Check sheet for the modelled part. Datum: model origin and axes. Units: mm. Face numbers are marked on the shaded views. Coordinates: 2 decimals unless noted, no trailing zeros. Loops run counter-clockwise (first coordinate to the right, second up) from the corner with the lowest first, then second, coordinate; pieces in that order, holes last. Notation, with made-up numbers: M 76,85.25 L 82,85.25 A8 ccw 82,95.25 Z; hole C 25.5,14.25 d6. An arc over 180 degrees is marked long. Answer in a Markdown table with one row per item. Add a question column.
```python
from build123d import *

# Parameters (mm, degrees)
SKETCH_1_R                = 60
EXTRUDE_1_DEPTH           = 10
SKETCH_4_R                = 30
CUT_EXTRUDE_1_DEPTH       = 86.440037453
HOLE_WIZARD_1_D           = 4.5
HOLE_WIZARD_1_CBORE_D     = 8
HOLE_WIZARD_1_CBORE_DEPTH = 4.6
PATTERN_CIRCULAR_1_COUNT  = 16
HOLE_WIZARD_2_D           = 5.5
HOLE_WIZARD_2_CBORE_D     = 10
HOLE_WIZARD_2_CBORE_DEPTH = 5.7
PATTERN_CIRCULAR_2_COUNT  = 10


with BuildPart() as part:
    # 草图1 → 凸台-拉伸1 (new body)
    with BuildSketch(Plane.XY):
        Circle(SKETCH_1_R)
    extrude(amount=EXTRUDE_1_DEPTH)

    # 草图4 → 切除-拉伸1 (cut, through all)
    with BuildSketch(Plane.XY.offset(10)):
        Circle(SKETCH_4_R)
    extrude(amount=-CUT_EXTRUDE_1_DEPTH, mode=Mode.SUBTRACT)

    # 打孔尺寸(%根据)内六角圆柱头螺钉的类型1 (through all)
    with Locations(Plane.XY.offset(10)):
        with Locations((0, 38.5)):
            hole_wizard_1 = CounterBoreHole(HOLE_WIZARD_1_D / 2, HOLE_WIZARD_1_CBORE_D / 2, HOLE_WIZARD_1_CBORE_DEPTH)

    # 阵列(圆周)1: 打孔尺寸(%根据)内六角圆柱头螺钉的类型1 ×16 about axis
    pattern_circular_1_axis = Axis((0, 0, 0), (0, 0, 1))
    for i in range(1, PATTERN_CIRCULAR_1_COUNT):
        add(hole_wizard_1.rotate(pattern_circular_1_axis, i * 360 / PATTERN_CIRCULAR_1_COUNT), mode=Mode.SUBTRACT)

    # 打孔尺寸(%根据)内六角圆柱头螺钉的类型2 (through all)
    with Locations(Plane(origin=(0, 0, 0), x_dir=(-1, 0, 0), z_dir=(0, 0, -1))):
        with Locations((0, 52.5)):
            hole_wizard_2 = CounterBoreHole(HOLE_WIZARD_2_D / 2, HOLE_WIZARD_2_CBORE_D / 2, HOLE_WIZARD_2_CBORE_DEPTH)

    # 阵列(圆周)2: 打孔尺寸(%根据)内六角圆柱头螺钉的类型2 ×10 about axis
    pattern_circular_2_axis = Axis((0, 0, 0), (0, 0, 1))
    for i in range(1, PATTERN_CIRCULAR_2_COUNT):
        add(hole_wizard_2.rotate(pattern_circular_2_axis, i * 360 / PATTERN_CIRCULAR_2_COUNT), mode=Mode.SUBTRACT)


solid = part.part
```
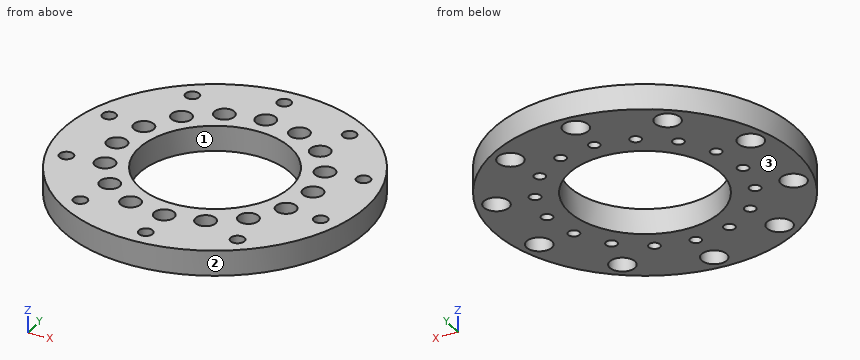
Q1. Mould release check, pull along Y, two halves, no side actions. Record for the marked faces 1, 2 and 3: released by +Y, released by -Y, zero draft, split by the parting line, or undercut.
Q2. Cross-section at C-C (y = -52.5). Record the cut outline in (x, z), plus the area to 3 significant figures.
Q3. Thickness scan on L1, parallel to Y at x = 0, z = 8.9; L2, parallel to Y at x = 0, z = 1.65; L3, parallel to Y at x = 51.5, z = 2.25. Record the ranges inside material, lowest first.
Q4. Go/stop test with flat-tipped pins: pin 1 (6 mm diameter, centred on y = -0.5, z = 9, fed in from +X); pin 2 (3 mm diameter, centred on x = 25.5, z = 4.5, fed in from -Y); pin 3 (1 mm diameter, centred on x = -42, z = 3.5, fed in from +Y); pin 4 (3.5 mm diameter, centred on x = 27.22, y = 27.22, fed in from +Z). Record where each tip stops, or that it passes through.
Q5. Cross-section at B-B (x = 0). Count the separate pieces of the cut face and the enclosed holes in it, plus the area to 4 significant figures.
Q6. Cross-section at A-A (y = 0). Record the cut outline in (x, z), plus the area to 3 significant figures.
Answer key:
| question | item | result |
|---|---|---|
| 1 | face 1 | undercut |
| 1 | face 2 | split by the parting line |
| 1 | face 3 | zero draft |
| 2 | outline | M -29.05,0 L -5,0 L -5,5.7 L -2.75,5.7 L -2.75,10 L -29.05,10 Z; M 2.75,5.7 L 5,5.7 L 5,0 L 29.05,0 L 29.05,10 L 2.75,10 Z |
| 2 | area | 500 mm^2 |
| 3 | L1 | -60 to -55.25, -49.75 to -42.5, -34.5 to -30, 30 to 34.5, 42.5 to 49.75, 55.25 to 60 |
| 3 | L2 | -60 to -57.5, -47.5 to -40.75, -36.25 to -30, 30 to 36.25, 40.75 to 47.5, 57.5 to 60 |
| 3 | L3 | -30.79 to -20.97, -11.48 to 11.48, 20.97 to 30.79 |
| 4 | pin 1 | x = 60 |
| 4 | pin 2 | y = -54.99 |
| 4 | pin 3 | y = 43.33 |
| 4 | pin 4 | through |
| 5 | separate pieces | 6 |
| 5 | enclosed holes | 0 |
| 5 | area | 316.5 mm^2 |
| 6 | outline | M -60,0 L -40.75,0 L -40.75,5.4 L -42.5,5.4 L -42.5,10 L -60,10 Z; M -36.25,0 L -30,0 L -30,10 L -34.5,10 L -34.5,5.4 L -36.25,5.4 Z; M 30,0 L 36.25,0 L 36.25,5.4 L 34.5,5.4 L 34.5,10 L 30,10 Z; M 40.75,0 L 60,0 L 60,10 L 42.5,10 L 42.5,5.4 L 40.75,5.4 Z |
| 6 | area | 478 mm^2 |
